```python
from build123d import *

# Parameters (mm, degrees)
SKETCH_2_W        = 20
SKETCH_2_H        = 20
SKETCH_2_R        = 1.6
EXTRUDE_433_DEPTH = 1.5
SKETCH_3_R        = 3
SKETCH_3_R_2      = 1.6
EXTRUDE_659_DEPTH = 5
CHAMFER_1_SIZE    = 1.5


with BuildPart() as part:
    # Эскиз2 → Extrude 433 (new body)
    with BuildSketch(Plane.XY):
        Rectangle(SKETCH_2_W, SKETCH_2_H)
        Circle(SKETCH_2_R, mode=Mode.SUBTRACT)
    extrude(amount=EXTRUDE_433_DEPTH)

    # Эскиз3 → Extrude 659 (add)
    with BuildSketch(Plane.XY.offset(1.5)):
        with Locations(Location((0, 0, 0), (0, 0, 180))):
            Circle(SKETCH_3_R)
        Circle(SKETCH_3_R_2, mode=Mode.SUBTRACT)
    extrude(amount=EXTRUDE_659_DEPTH)

    # Фаска1
    chamfer_1_edges = [part.edges().sort_by_distance(p)[0] for p in [
        (-1.6, 0, 0),
    ]]
    chamfer(chamfer_1_edges, length=CHAMFER_1_SIZE)


solid = part.part
```
Source: CAD feature listing. Evaluate the final solid. Frame: model axes, mm. A direction names the side the tool comes from. Give positions to 0.01 mm unless a question says otherwise; leave off trailing zeros. Write each loop counter-clockwise with the first axis right and the second up, starting at its lowest first coordinate (ties: lowest second). Pieces come first, ordered by that corner, then holes.
1. Section query D-D (y = 4.25). Return the cut outline in (x, z).
2. Access query for faces 5 (the face through (-2.4, 2.4, 1.5)), 6 (the face through (0, -10, 1)). Directions: +Z, -Z, +X, -X, +Y, -Y. A direction counts if a zero-diameter tool reaches every point of the face in a straight line with its end or side. Return the directions, or none.
3. Pull-direction query (Y, two-part tool) for faces 1 (the face through (-1.27, -0.97, 3.96)), 2 (the face through (-2.4, 2.4, 0)), 3 (the face through (0, 10, 1)), 4 (the face through (-2.86, -0.9, 3.96)); classes: +Y half, -Y half, draft (parallel to the pull), parting line (faces both ways), or undercut.
4. First-contact query: pin 1 (2 mm diameter, centred on y = 3.5, z = 4, fed in from +X); pin 2 (2 mm diameter, centred on x = 3, y = -5.5, fed in from +Z). Flat tips, straight axial feed; report the tip coordinate or a pass-through.
5. Material intervals for line 1 along Y through (x, z) = (0, 5.25); line 2 along Z through (x, y) = (-1.5, 5.75); line 3 along X through (y, z) = (-1, 5.25), sorted ascending.
6. Section query A-A (y = 0). Return the cut outline in (x, z).
7. Section query C-C (z = 1). Return the cut outline in (x, y).
Output values:
1. outline: (-10, 0) - (10, 0) - (10, 1.5) - (-10, 1.5) - close
2. face 5: +Z
2. face 6: +Z, -Z, +X, -X, -Y
3. face 1: undercut
3. face 2: draft
3. face 3: +Y half
3. face 4: parting line
4. pin 1: stops at x = 1.66
4. pin 2: stops at z = 1.5
5. line 1: y = -3 to -1.6, 1.6 to 3
5. line 2: z = 0 to 1.5
5. line 3: x = -2.83 to -1.25, 1.25 to 2.83
6. outline: (-10, 0) - (-3.1, 0) - (-1.6, 1.5) - (-1.6, 6.5) - (-3, 6.5) - (-3, 1.5) - (-10, 1.5) - close; (1.6, 1.5) - (3.1, 0) - (10, 0) - (10, 1.5) - (3, 1.5) - (3, 6.5) - (1.6, 6.5) - close
7. outline: (-10, -10) - (10, -10) - (10, 10) - (-10, 10) - close; hole circle Ø4.2 at (0, 0)
